Build history of the part. All positions in model axes, mm. A direction names the side the tool comes from. Give positions to 0.01 mm unless a question says otherwise; leave off trailing zeros. Order: outer loops, then holes, each group sorted by start corner. A loop starts at its lowest first (then second) coordinate and runs counter-clockwise, first axis right, second up. Notation, with made-up numbers: M 47.5,6.25 L 95.5,6.25 A22 ccw 95.5,27.25 Z; hole C -8,65 d2. An arc over 180 degrees is marked long. One line per item, written item: value.
from build123d import *

# Parameters (mm, degrees)
SKETCH1_W           = 17.1
SKETCH1_H           = 31.8
BOSS_EXTRUDE1_DEPTH = 1.2
SKETCH2_W           = 13.399731937
SKETCH2_H           = 1.34283028
SKETCH2_W_2         = 1.999959991
SKETCH2_H_2         = 17.228226777
BOSS_EXTRUDE2_DEPTH = 2
SKETCH3_W           = 8.02841082
SKETCH3_H           = 3.314219413
BOSS_EXTRUDE3_DEPTH = 5


with BuildPart() as part:
    # Sketch1 → Boss-Extrude1 (new body)
    with BuildSketch(Plane(origin=(0, 0, 0), x_dir=(1, 0, 0), z_dir=(0, 1, 0))):
        with Locations((8.55, -15.9)):
            Rectangle(SKETCH1_W, SKETCH1_H)
    extrude(amount=BOSS_EXTRUDE1_DEPTH)

    # Sketch2 → Boss-Extrude2 (add)
    with BuildSketch(Plane(origin=(0, 1.2, 0), x_dir=(1, 0, 0), z_dir=(0, 1, 0))):
        with Locations((8.478572857, -1.557429781)):
            Rectangle(SKETCH2_W, SKETCH2_H)
        with Locations((15.035584542, -20.699903977)):
            Rectangle(SKETCH2_W_2, SKETCH2_H_2)
    extrude(amount=BOSS_EXTRUDE2_DEPTH)

    # Sketch3 → Boss-Extrude3 (add)
    with BuildSketch(Plane(origin=(0, 1.2, 0), x_dir=(1, 0, 0), z_dir=(0, 1, 0))):
        with Locations((3.335818596, -27.856903659)):
            Rectangle(SKETCH3_W, SKETCH3_H)
    extrude(amount=BOSS_EXTRUDE3_DEPTH)


solid = part.part
1) Mould opens along X. For faces 1 (the face through (17.1, 1, 16)), 2 (the face through (3, 6.2, 28)), 3 (the face through (7.35, 4, 28)) say: released by +X, released by -X, zero draft, split by the parting line, or undercut.
Check values:
face 1: released by +X
face 2: zero draft
face 3: undercut
2) Saw through at B-B, the plane z = 19. Write the cut outline in (x, y), then the cut area to 3 significant figures.
Check values:
outline: M 0,0 L 17.1,0 L 17.1,1.2 L 16.04,1.2 L 16.04,3.2 L 14.04,3.2 L 14.04,1.2 L 0,1.2 Z
area: 24.5 mm^2
3) Tool access for faces 4 (the face through (15, 2, 12.086)), 5 (the face through (3, 4, 26.2)), 6 (the face through (3, 4, 29.514)), 7 (the face through (15, 2, 29.314)), 8 (the face through (8, 2, 0.886)): list every direction of +Z, -Z, +X, -X, +Y, -Y with a clear straight run to the whole face (end or side of a thin tool).
Check values:
face 4: +X, -X, +Y
face 5: -X, +Y
face 6: +Z, +X, -X, +Y
face 7: +Z, +X, +Y
face 8: -Z, +X, -X, +Y
4) Saw through at A-A, the plane x = 10. Write the cut outline in (y, z).
Check values:
outline: M 0,0 L 1.2,0 L 1.2,0.89 L 3.2,0.89 L 3.2,2.23 L 1.2,2.23 L 1.2,31.8 L 0,31.8 Z
5) Drill centre lines: probe 1 along Z at (x, y) = (4.75, 2.5); probe 2 along Y at (x, z) = (2, 8); probe 3 along X at (y, z) = (2.25, 19). Where is each one in solid material? Low to high. Write a range as from..to.
Check values:
probe 1: 0.89..2.23, 26.2..29.51
probe 2: 0..1.2
probe 3: 14.04..16.04
6) Pin check, flat tips, straight feed: pin 1 (1.5 mm diameter, centred on x = 10, z = 1.5, fed in from +Y); pin 2 (2 mm diameter, centred on y = 2.5, z = 18.5, fed in from -X); pin 3 (1.5 mm diameter, centred on x = 3.5, z = 20.5, fed in from +Y). Stop position of each tip, or through.
Check values:
pin 1: y = 3.2
pin 2: x = 14.04
pin 3: y = 1.2
7) Saw through at D-D, the plane x = 6.5. Write the cut outline in (y, z).
Check values:
outline: M 0,0 L 1.2,0 L 1.2,0.89 L 3.2,0.89 L 3.2,2.23 L 1.2,2.23 L 1.2,26.2 L 6.2,26.2 L 6.2,29.51 L 1.2,29.51 L 1.2,31.8 L 0,31.8 Z
8) Saw through at C-C, the plane y = 5.25. Write the cut outline in (x, z), then the cut area to 3 significant figures.
Check values:
outline: M -0.68,26.2 L 7.35,26.2 L 7.35,29.51 L -0.68,29.51 Z
area: 26.6 mm^2
